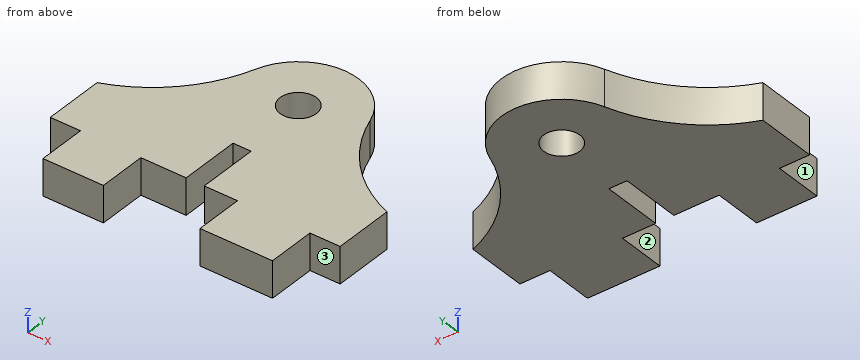
from build123d import *

# Parameters (mm, degrees)
SKETCH1_R           = 1.5
SKETCH1_R_2         = 1
BOSS_EXTRUDE1_DEPTH = 3
SKETCH2_W           = 21.215315346
SKETCH2_H           = 10.620784377
CUT_EXTRUDE1_DEPTH  = 4
SKETCH3_W           = 2.5
SKETCH3_H           = 4
CUT_EXTRUDE2_DEPTH  = 10
SKETCH4_W           = 2.5
SKETCH4_H           = 4
BOSS_EXTRUDE2_DEPTH = 3
SKETCH5_W           = 2.5
SKETCH5_H           = 5.5
BOSS_EXTRUDE3_DEPTH = 3
SKETCH6_W           = 1.5
SKETCH6_H           = 10
CUT_EXTRUDE3_DEPTH  = 5


with BuildPart() as part:
    # Sketch1 → Boss-Extrude1 (new body)
    with BuildSketch(Plane.XY):
        with BuildLine():
            Line((-1.25, -11), (-7, -11))
            Line((-7, -11), (-7, -15))
            Line((-7, -15), (-12, -15))
            Line((-12, -15), (-12, -11))
            Line((-12, -11), (-12, -6))
            ThreePointArc((-12, -6), (-7.512319363, -3.05842228), (-4.755323166, 1.544960058))
            ThreePointArc((-4.755323166, 1.544960058), (0, 5), (4.755323166, 1.544960058))
            ThreePointArc((4.755323166, 1.544960058), (7.512319363, -3.05842228), (12, -6))
            Line((12, -6), (12, -22.5))
            ThreePointArc((12, -22.5), (11.267766953, -24.267766953), (9.5, -25))
            Line((9.5, -25), (8.5, -25))
            ThreePointArc((8.5, -25), (6.732233047, -24.267766953), (6, -22.5))
            Line((6, -22.5), (6, -11))
            Line((6, -11), (1.25, -11))
            Line((1.25, -11), (1.25, -5.5))
            Line((1.25, -5.5), (-1.25, -5.5))
            Line((-1.25, -5.5), (-1.25, -11))
        make_face()
        Circle(SKETCH1_R, mode=Mode.SUBTRACT)
        with Locations((9, -22)):
            Circle(SKETCH1_R_2, mode=Mode.SUBTRACT)
    extrude(amount=BOSS_EXTRUDE1_DEPTH)

    # Sketch2 → Cut-Extrude1 (cut, through all)
    with BuildSketch(Plane.XY.offset(3)):
        with Locations((3.607657673, -20.310392189)):
            Rectangle(SKETCH2_W, SKETCH2_H)
    extrude(amount=-CUT_EXTRUDE1_DEPTH, mode=Mode.SUBTRACT)

    # Sketch3 → Cut-Extrude2 (cut)
    with BuildSketch(Plane.XY.offset(3)):
        with Locations((10.75, -13)):
            Rectangle(SKETCH3_W, SKETCH3_H)
        with Locations((-10.75, -13)):
            Rectangle(SKETCH3_W, SKETCH3_H)
    extrude(amount=-CUT_EXTRUDE2_DEPTH, mode=Mode.SUBTRACT)

    # Sketch4 → Boss-Extrude2 (add)
    with BuildSketch(Plane.XY.offset(3)):
        with Locations((-5.75, -13)):
            Rectangle(SKETCH4_W, SKETCH4_H)
        with Locations((4.75, -13)):
            Rectangle(SKETCH4_W, SKETCH4_H)
    extrude(amount=-BOSS_EXTRUDE2_DEPTH)

    # Sketch5 → Boss-Extrude3 (add)
    with BuildSketch(Plane(origin=(0, 0, 0), x_dir=(-1, 0, 0), z_dir=(0, 0, -1))):
        with Locations((0, -8.25)):
            Rectangle(SKETCH5_W, SKETCH5_H)
    extrude(amount=-BOSS_EXTRUDE3_DEPTH)

    # Sketch6 → Cut-Extrude3 (cut)
    with BuildSketch(Plane(origin=(0, 0, 0), x_dir=(-1, 0, 0), z_dir=(0, 0, -1))):
        with Locations((0, -11)):
            Rectangle(SKETCH6_W, SKETCH6_H)
    extrude(amount=-CUT_EXTRUDE3_DEPTH, mode=Mode.SUBTRACT)


solid = part.part
Build history of the part. All positions in model axes, mm. Face numbers are marked on the shaded views. A direction names the side the tool comes from. Round coordinates to 2 decimals unless told otherwise and drop trailing zeros. Order: outer loops, then holes, each group sorted by start corner. A loop starts at its lowest first (then second) coordinate and runs counter-clockwise, first axis right, second up. Notation, with made-up numbers: M 13.5,37.25 L 55.5,37.25 A11 ccw 55.5,50.25 Z; hole C -8,-21 d7. An arc over 180 degrees is marked long. Use CSV: the item, a comma, the result in double quotes. Start each with the question number.
(1) Cut at A-A on z = 1. List the corners of the cut face in (x, y).
(2) Cut at C-C on y = 0. List the corners of the cut face in (x, z).
(3) Cut at B-B on x = 0. List the corners of the cut face in (y, z), then the cut area to 3 significant figures.
(4) Flat gauge pins, fed straight in: P1, Ø1.2, axis at x = -11.5, z = 1.5, coming from the -Y side; P2, Ø1.5, axis at x = -6, z = 1, coming from the +Y side; P3, Ø1.5, axis at y = -12, z = 1.5, coming from the +X side. Where does each tip first touch, or does it go through?
(5) Cut at D-D on x = 4. List the corners of the cut face in (y, z), then the cut area to 3 significant figures.
(6) Drill centre lines: probe 1 along Y at (x, z) = (0, 1.4); probe 2 along X at (y, z) = (-7, 1.3); probe 3 along Y at (x, z) = (0.5, 1.7). Where is each one in solid material? Low to high.
(7) Tool access for the marked faces 1, 2 and 3: list every direction of +Z, -Z, +X, -X, +Y, -Y with a clear straight run to the whole face (end or side of a thin tool).
Findings:
1,outline,"M -12,-11 L -9.5,-11 L -9.5,-15 L -4.5,-15 L -4.5,-11 L -0.75,-11 L -0.75,-6 L 0.75,-6 L 0.75,-11 L 3.5,-11 L 3.5,-15 L 9.5,-15 L 9.5,-11 L 12,-11 L 12,-6 A12 cw 4.76,1.54 A5 ccw -4.76,1.54 A12 cw -12,-6 Z; hole C 0,0 d3"
2,outline,"M -5.38,0 L -1.5,0 L -1.5,3 L -5.38,3 Z; M 1.5,0 L 5.38,0 L 5.38,3 L 1.5,3 Z"
3,outline,"M -6,0 L -1.5,0 L -1.5,3 L -6,3 Z; M 1.5,0 L 5,0 L 5,3 L 1.5,3 Z"
3,area,"24.0 mm^2"
4,P1,"stops at y = -11"
4,P2,"stops at y = 0.27"
4,P3,"stops at x = 9.5"
5,outline,"M -15,0 L 3,0 L 3,3 L -15,3 Z"
5,area,"54.0 mm^2"
6,probe 1,"y = -6 to -1.5, 1.5 to 5"
6,probe 2,"x = -12 to -0.75, 0.75 to 12"
6,probe 3,"y = -6 to -1.41, 1.41 to 4.97"
7,face 1,"+Z, -Z, -X, -Y"
7,face 2,"+Z, -Z, -Y"
7,face 3,"+Z, -Z, +X, -Y"
